Geometry check sheet. Reference: drawing and pictorial views, mm from the part's lowest x, y, z. Coordinates: 2 decimals unless noted, no trailing zeros. Write each loop counter-clockwise with the first axis right and the second up, starting at its lowest first coordinate (ties: lowest second). Pieces come first, ordered by that corner, then holes. Notation, with made-up numbers: (-31, 15) -> (-10, 15) arc R18 ccw to (-10, 32) -> close; hole circle Ø4 at (72, 65.25). An arc over 180 degrees is marked (long way). Answer in a Markdown table with one row per item.
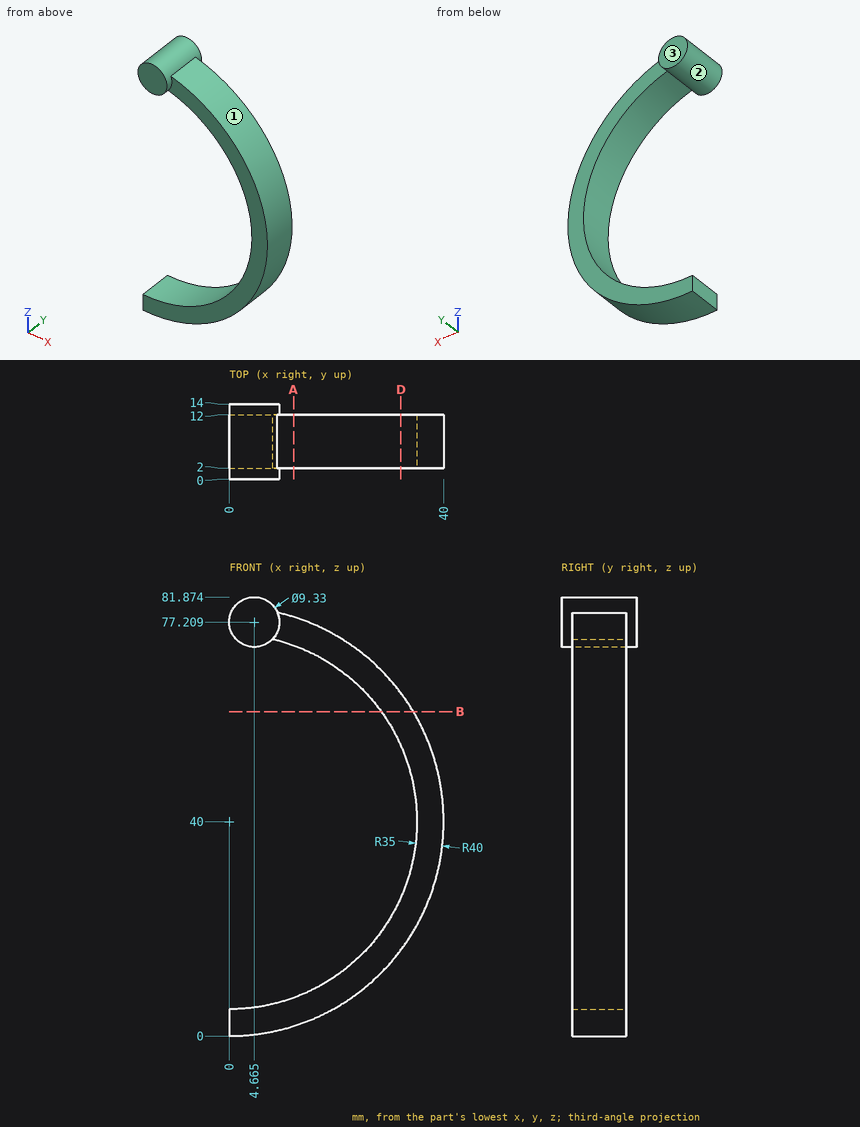
1. Section check B-B, the plane z = 60.5. Record the boundary of the cut face in (x, y).
Geometry says:
| item | result |
|---|---|
| outline | (28.37, 2) -> (34.35, 2) -> (34.35, 12) -> (28.37, 12) -> close |
2. Mould release check, pull along Z, two halves, no side actions. Record for the marked faces 1, 2 and 3: released by +Z, released by -Z, zero draft, split by the parting line, or undercut.
Geometry says:
| item | result |
|---|---|
| face 1 | split by the parting line |
| face 2 | undercut |
| face 3 | zero draft |
3. Thickness scan on line 1 (Z direction, x = 5, y = 1.5) (1 decimal); line 2 (Z direction, x = 31, y = 8.75); line 3 (Y direction, x = 34, z = 19). Record the ranges inside material, lowest first. Write a range as from..to.
Geometry says:
| item | result |
|---|---|
| line 1 | 72.6..81.9 |
| line 2 | 14.72..23.75, 56.25..65.28 |
| line 3 | 2..12 |
4. Section check D-D, the plane x = 32. Record the boundary of the cut face in (y, z).
Geometry says:
| item | result |
|---|---|
| outline | (2, 16) -> (12, 16) -> (12, 25.82) -> (2, 25.82) -> close; (2, 54.18) -> (12, 54.18) -> (12, 64) -> (2, 64) -> close |
5. Depth check by flat-ended pin: P1, Ø8, axis at y = 7.5, z = 14, coming from the +X side; P2, Ø1.5, axis at x = 30, y = 3.5, coming from the -Z side (1 decimal); P3, Ø2, axis at y = 3, z = 60.5, coming from the +X side (1 decimal). Enter the tip coordinate at first touch or a pass-through.
Geometry says:
| item | result |
|---|---|
| P1 | x = 33.41 |
| P2 | z = 12.7 |
| P3 | x = 34.9 |
6. Section check A-A, the plane x = 12. Record the boundary of the cut face in (y, z).
Geometry says:
| item | result |
|---|---|
| outline | (2, 1.84) -> (12, 1.84) -> (12, 7.12) -> (2, 7.12) -> close; (2, 72.88) -> (12, 72.88) -> (12, 78.16) -> (2, 78.16) -> close |
